The model under review builds one solid part; all positions refer to its coordinate system, in mm. A direction names the side the tool comes from. Round coordinates to 2 decimals unless told otherwise and drop trailing zeros. Loops run counter-clockwise (first coordinate to the right, second up) from the corner with the lowest first, then second, coordinate; pieces in that order, holes last. Notation, with made-up numbers: M -28,86 L -1,86 A19 cw -1,101 Z; hole C -34,20.25 d1. An arc over 180 degrees is marked long. Return JSON: item names as keys, results as strings. Group by question number.
Q1. Draft analysis for pull direction X (two halves, no side actions). For faces 4 (the face through (12.02, 29.116, 17.206)), 5 (the face through (14, 43.2, 18)), 6 (the face through (19.3, 33, 20)), state which applies: pulls with the +X half, pulls with the -X half, needs draft (parallel to the pull), parting line crosses it, or undercut.
Q2. To check wall thickness, follow line 1 along X through (y, z) = (25, 26); line 2 along X through (y, z) = (25, 0); line 3 along X through (y, z) = (12, 11). State the ranges of each line that lie inside material, in increasing order.
Q3. Consider section C-C (y = 18.5). Count the separate pieces of the cut face and the enclosed holes in it, and give its area (3 significant figures).
Q4. Clearance check with flat-ended pins moving along their axes: pin 1 Ø1.5 at (x, y) = (13.5, 35) entering from -Z; pin 2 Ø5 at (x, y) = (11, 47.5) entering from -Z; pin 3 Ø0.8 at (x, z) = (-13.5, 18.5) entering from +Y. State where each tip first meets the part, or that it passes through.
Q5. For faces 1 (the face through (-16.816, 29.116, 17.206)), 2 (the face through (-13.61, 42.46, 12.82)), 3 (the face through (-0.501, 13.501, -16.062)), list the 3-axis set-ups (+Z, -Z, +X, -X, +Y, -Y) from which the entire face can be reached by the end or side of a thin tool; tool diameter is ignored.
Q6. Consider section B-B (z = -14). State the section outline as (x, y) points, and give its area (3 significant figures).
Q7. Consider section A-A (x = 0). State the section outline as (y, z) points, and give its area (3 significant figures).
Q8. Consider section D-D (x = -6). State the section outline as (y, z) points.
from build123d import *

# Parameters (mm, degrees)
EXTRUDE_1_DEPTH       = 1.68
SKETCH_2_R            = 14.75
EXTRUDE_3_DEPTH       = 5
EXTRUDE_4_DEPTH       = 1.68
EXTRUDE_5_DEPTH       = 40
CUT_EXTRUDE_1_DEPTH   = 30
FILLET_1_R            = 10
SKETCH_6_R            = 20
EXTRUDE_6_DEPTH       = 9.9
SKETCH_7_R            = 13
EXTRUDE_7_DEPTH       = 11.3
EXTRUDE_8_DEPTH       = 19.3
FILLET_2_R            = 1
SKETCH_9_W            = 67.955976502
SKETCH_9_H            = 118.115360496
CUT_EXTRUDE_1_2_DEPTH = 6.68


with BuildPart() as part:
    # Sketch 1 → Extrude 1 (new body)
    with BuildSketch(Plane(origin=(0, 0, 0), x_dir=(1, 0, 0), z_dir=(0, 1, 0))):
        with BuildLine():
            ThreePointArc((-21.5, 23.6), (-19.6254834, 28.1254834), (-15.1, 30))
            Line((-15.1, 30), (15.1, 30))
            ThreePointArc((15.1, 30), (19.6254834, 28.1254834), (21.5, 23.6))
            Line((21.5, 23.6), (21.5, -23.6))
            ThreePointArc((21.5, -23.6), (19.6254834, -28.1254834), (15.1, -30))
            Line((15.1, -30), (-15.1, -30))
            ThreePointArc((-15.1, -30), (-19.6254834, -28.1254834), (-21.5, -23.6))
            Line((-21.5, -23.6), (-21.5, 23.6))
        make_face()
        with BuildLine():
            ThreePointArc((-18.2, -23.95), (-15, -27.15), (-11.8, -23.95))
            Line((-11.8, -23.95), (-11.8, -21.05))
            ThreePointArc((-11.8, -21.05), (-15, -17.85), (-18.2, -21.05))
            Line((-18.2, -21.05), (-18.2, -23.95))
        make_face(mode=Mode.SUBTRACT)
        with BuildLine():
            ThreePointArc((18.2, -21.05), (15, -17.85), (11.8, -21.05))
            Line((11.8, -21.05), (11.8, -23.95))
            ThreePointArc((11.8, -23.95), (15, -27.15), (18.2, -23.95))
            Line((18.2, -23.95), (18.2, -21.05))
        make_face(mode=Mode.SUBTRACT)
        with BuildLine():
            ThreePointArc((18.2, 23.95), (15, 27.15), (11.8, 23.95))
            Line((11.8, 23.95), (11.8, 21.05))
            ThreePointArc((11.8, 21.05), (15, 17.85), (18.2, 21.05))
            Line((18.2, 21.05), (18.2, 23.95))
        make_face(mode=Mode.SUBTRACT)
        with BuildLine():
            ThreePointArc((-18.2, 21.05), (-15, 17.85), (-11.8, 21.05))
            Line((-11.8, 21.05), (-11.8, 23.95))
            ThreePointArc((-11.8, 23.95), (-15, 27.15), (-18.2, 23.95))
            Line((-18.2, 23.95), (-18.2, 21.05))
        make_face(mode=Mode.SUBTRACT)
    extrude(amount=EXTRUDE_1_DEPTH)

    # Sketch 2 → Extrude 3 (add)
    with BuildSketch(Plane(origin=(0, 1.68, 0), x_dir=(1, 0, 0), z_dir=(0, 1, 0))):
        Circle(SKETCH_2_R)
    extrude(amount=EXTRUDE_3_DEPTH)

    # Sketch 3 → Extrude 4 (add)
    with BuildSketch(Plane(origin=(0, 6.68, 0), x_dir=(1, 0, 0), z_dir=(0, 1, 0))):
        with BuildLine():
            Line((-14.4, -10.377981499), (-14.4, -50))
            Line((-14.4, -50), (14.4, -50))
            Line((14.4, -50), (14.4, -10.377981499))
            ThreePointArc((14.4, -10.377981499), (0, 17.75), (-14.4, -10.377981499))
        make_face()
    extrude(amount=EXTRUDE_4_DEPTH)

    # Sketch 4 → Extrude 5 (add)
    with BuildSketch(Plane(origin=(0, 8.36, 0), x_dir=(1, 0, 0), z_dir=(0, 1, 0))):
        with BuildLine():
            Line((-14.4, -50), (-12.72, -50))
            Line((-12.72, -50), (-12.72, -9.820717896))
            ThreePointArc((-12.72, -9.820717896), (0, 16.07), (12.72, -9.820717896))
            Line((12.72, -9.820717896), (12.72, -50))
            Line((12.72, -50), (14.4, -50))
            Line((14.4, -50), (14.4, -10.377981499))
            ThreePointArc((14.4, -10.377981499), (0, 17.75), (-14.4, -10.377981499))
            Line((-14.4, -10.377981499), (-14.4, -50))
        make_face()
    extrude(amount=EXTRUDE_5_DEPTH)

    # Sketch 5 → Cut-Extrude 1 (cut, symmetric)
    with BuildSketch(Plane(origin=(0, 0, 0), x_dir=(0, 0, -1), z_dir=(1, 0, 0))):
        Polygon((24.967425324, 5.782574676), (-12.45, 43.2), (-33.035504508, 43.2), (-22.754734371, 4.83164351), (-61.391767423, -5.521118294), (-85.164519421, 83.2), (4.118542495, 83.2), (53.251696571, 34.066845924), align=None)
    extrude(amount=CUT_EXTRUDE_1_DEPTH, both=True, mode=Mode.SUBTRACT)

    # Fillet 1
    fillet_1_edges = [part.edges().sort_by_distance(p)[0] for p in [
        (-13.56, 43.2, 33.035504508),
        (-13.56, 43.2, 12.45),
        (13.56, 43.2, 12.45),
        (13.56, 43.2, 33.035504508),
    ]]
    fillet(fillet_1_edges, radius=FILLET_1_R)



with BuildPart() as body_2:
    # Sketch 6 → Extrude 6 (new body, symmetric)
    with BuildSketch(Plane(origin=(0, 0, 0), x_dir=(0, 0, -1), z_dir=(1, 0, 0))):
        with Locations((-20.003250779, 33.2)):
            Circle(SKETCH_6_R)
    extrude(amount=EXTRUDE_6_DEPTH, both=True)

    # Sketch 7 → Extrude 7 (add, symmetric)
    with BuildSketch(Plane(origin=(0, 0, 0), x_dir=(0, 0, -1), z_dir=(1, 0, 0))):
        with Locations((-20.003250779, 33.2)):
            Circle(SKETCH_7_R)
    extrude(amount=EXTRUDE_7_DEPTH, both=True)


with BuildPart() as part_1:
    add(part.part)

    add(body_2.part)  # Extrude 8 merges body 2
    # Sketch 8 → Extrude 8 (add, symmetric)
    with BuildSketch(Plane(origin=(0, 0, 0), x_dir=(0, 0, -1), z_dir=(1, 0, 0))):
        Polygon((-24.693031377, 29.932591556), (-19.518482361, 27.504826642), (-14.828701763, 30.772235086), (-15.313470181, 36.467408444), (-20.488019197, 38.895173358), (-25.177799795, 35.627764914), align=None)
    extrude(amount=EXTRUDE_8_DEPTH, both=True)

    # Fillet 2
    fillet_2_edges = [part_1.edges().sort_by_distance(p)[0] for p in [
        (-9.9, 33.2, 40.003250779),
        (9.9, 33.2, 40.003250779),
    ]]
    fillet(fillet_2_edges, radius=FILLET_2_R)

    # Sketch 9 → Cut-Extrude 1 2 (cut)
    with BuildSketch(Plane.XZ):
        Rectangle(SKETCH_9_W, SKETCH_9_H)
    extrude(amount=-CUT_EXTRUDE_1_2_DEPTH, mode=Mode.SUBTRACT)


solid = part_1.part
Values:
{
 "1": {"face 4": "undercut", "face 5": "needs draft", "face 6": "pulls with the +X half"},
 "2": {"line 1": "x = -14.4 to -12.72, -11.3 to 11.3, 12.72 to 14.4", "line 2": "x = -17.75 to -16.07, 16.07 to 17.75", "line 3": "x = -14.4 to -12.72, 12.72 to 14.4"},
 "3": {"separate pieces": "3", "enclosed holes": "0", "area": "673 mm2"},
 "4": {"pin 1": "stops at z = 7.43", "pin 2": "stops at z = 4.46", "pin 3": "stops at y = 43.2"},
 "5": {"face 1": "-X, -Y", "face 2": "-Z, -X, +Y", "face 3": "+Y"},
 "6": {"outline": "M -10.91,6.68 L 10.91,6.68 L 10.91,16.75 L 7.89,16.75 L 7.89,8.36 L -7.89,8.36 L -7.89,16.75 L -10.91,16.75 Z", "area": "87.4 mm2"},
 "7": {"outline": "M 6.68,-17.75 L 13,-17.75 L 14.68,-16.07 L 8.36,-16.07 L 8.36,23.7 L 6.68,23.25 Z; C 33.2,20 d40", "area": "1,340 mm2"},
 "8": {"outline": "M 6.68,-16.71 L 14.04,-16.71 L 15.84,-14.91 L 8.36,-14.91 L 8.36,23.7 L 6.68,23.25 Z; C 33.2,20 d40"}
}
